Part model, mm, in its own coordinate system. Face numbers are marked on the shaded views. A direction names the side the tool comes from. Give positions to 0.01 mm unless a question says otherwise; leave off trailing zeros. Write each loop counter-clockwise with the first axis right and the second up, starting at its lowest first coordinate (ties: lowest second). Pieces come first, ordered by that corner, then holes. Notation, with made-up numbers: M 61.5,89.5 L 116.5,89.5 A15 ccw 116.5,97.5 Z; hole C 65,-28 d9. An arc over 180 degrees is marked long. Answer as CSV lines item,"result". Start each with the question number.
Item 1: Wall check: L1, parallel to X at y = 7, z = 0; L2, parallel to Y at x = 9.5, z = -4.75; L3, parallel to X at y = 8.4, z = 0 (3 decimals). Give the ranges that are in metal, low to high. Write a range as from..to.
Item 2: Pin check, flat tips, straight feed: pin 1 (5 mm diameter, centred on x = 5.5, y = 3.5, fed in from +Z); pin 2 (1.5 mm diameter, centred on x = 7.5, z = 9.5, fed in from -Y); pin 3 (12.5 mm diameter, centred on x = 0, z = 0, fed in from +Y); pin 4 (6.5 mm diameter, centred on x = 0, z = 0, fed in from +Y). Stop position of each tip, or through.
Item 3: 3-axis set-ups, long thin cutter, end or side, ignore diameter. For the marked faces 1, 2 and 3: which of +Z, -Z, +X, -X, +Y, -Y reach the whole face in a straight line?
Item 4: Band-saw the part on A-A, the plane y = 6.5. List the corners of the cut face in (x, z), then the cut area to 3 significant figures.
from build123d import *
from build123d.topology import SkipClean

# Parameters (mm, degrees)
SKETCH1_R           = 12.7
BOSS_EXTRUDE1_DEPTH = 7.9375
SKETCH2_R           = 3.96875
CUT_EXTRUDE1_DEPTH  = 20.636290542
SKETCH5_R           = 8.255
SKETCH5_R_2         = 3.96875
BOSS_EXTRUDE2_DEPTH = 4.7625


with BuildPart() as part:
    # Sketch1 → Boss-Extrude1 (new body)
    with BuildSketch(Plane(origin=(0, 0, 0), x_dir=(1, 0, 0), z_dir=(0, 1, 0))):
        with Locations(Location((0, 0, 0), (0, 0, 270))):
            Circle(SKETCH1_R)
    extrude(amount=BOSS_EXTRUDE1_DEPTH)

    # Sketch2 → Cut-Extrude1 (cut, through all)
    with BuildSketch(Plane(origin=(0, 7.9375, 0), x_dir=(1, 0, 0), z_dir=(0, 1, 0))):
        with Locations(Location((0, 0, 0), (0, 0, 270))):
            Circle(SKETCH2_R)
    extrude(amount=-CUT_EXTRUDE1_DEPTH, mode=Mode.SUBTRACT)

    # Sketch4 → Cut-Revolve1 (revolve, cut)
    with BuildSketch(Plane(origin=(0, 0, 0), x_dir=(0, 0, -1), z_dir=(1, 0, 0))):
        with BuildLine():
            Line((-12.7, 6.9215), (-12.7, 1.016))
            ThreePointArc((-12.7, 1.016), (-11.2268, 3.96875), (-12.7, 6.9215))
        make_face()
    revolve(axis=Axis((0, 8.334375, 0), (0, -1, 0)), mode=Mode.SUBTRACT)

    # Sketch5 → Boss-Extrude2 (add, symmetric)
    with SkipClean():  # the faces are left unmerged after this step: merging them gives an invalid solid
        with BuildSketch(Plane(origin=(0, 3.937, 0), x_dir=(-1, 0, 0), z_dir=(0, -1, 0))):
            Circle(SKETCH5_R)
            with Locations(Location((0, 0, 0), (0, 0, 180))):
                Circle(SKETCH5_R_2, mode=Mode.SUBTRACT)
        extrude(amount=BOSS_EXTRUDE2_DEPTH, both=True)


solid = part.part
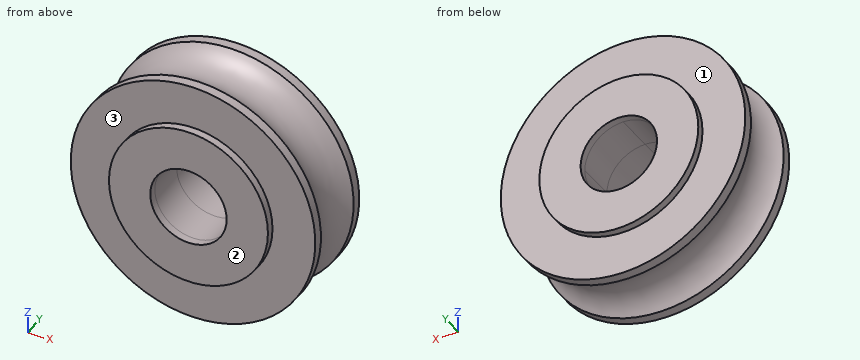
Output:
1,L1,"-12.7..-3.97, 3.97..12.7"
1,L2,"0..7.94"
1,L3,"-8.255..-3.969, 3.969..8.255"
2,pin 1,"z = 11.64"
2,pin 2,"y = 0"
2,pin 3,"y = 8.7"
2,pin 4,"through"
3,face 1,"+Y"
3,face 2,"+Z, -Z, +X, -X, -Y"
3,face 3,"-Y"
4,outline,"C 0,0 d24.46; hole C 0,0 d7.94"
4,area,"420 mm²"
